Geometry: final body of the model. Coordinates: model frame, mm. Face numbers are marked on the shaded views. A direction names the side the tool comes from. Give positions to 0.01 mm unless a question says otherwise; leave off trailing zeros. Write each loop counter-clockwise with the first axis right and the second up, starting at its lowest first coordinate (ties: lowest second). Pieces come first, ordered by that corner, then holes. Notation, with made-up numbers: (-10.5, -15.5) -> (34.5, -15.5) arc R17 ccw to (34.5, -11.5) -> close; hole circle Ø2 at (-33.5, 19). An arc over 180 degrees is marked (long way). Answer as a JSON object with one key per item and string values. Group by question number.
(1) Section query D-D on z = 3.5. Output: boundary loops of the cut face in (x, y), plus the area to 3 significant figures.
(2) Section query A-A on x = 12.7. Output: boundary loops of the cut face in (y, z), plus the area to 3 significant figures.
(3) Draft query along Z for the marked faces 3, 4 and 5. Return one class per face: +Z half, -Z half, draft (parallel to the pull), parting line (faces both ways), or undercut.
(4) Material intervals for probe 1 along X at (y, z) = (0.75, 0); probe 2 along Z at (x, y) = (12.5, -6.5); probe 3 along Y at (x, z) = (18.25, 4.5), sorted ascending.
(5) Section query B-B on z = 0. Output: boundary loops of the cut face in (x, y), plus the area to 3 significant figures.
(6) Section query C-C on x = 2.75. Output: boundary loops of the cut face in (y, z).
(7) Contact query for flat-ended pins moving along their axis: pin 1 Ø5 at (x, z) = (13, 0) entering from +Y; pin 2 Ø3.5 at (x, z) = (12.7, 0) entering from -Y; pin 3 Ø0.6 at (y, z) = (7, 6.5) entering from -X; pin 4 Ø0.9 at (y, z) = (-0.5, -6.5) entering from -X. Output: stop coordinate, or through.
(8) Set-up query: the marked faces 1 and 2. Return all of +Z, -Z, +X, -X, +Y, -Y with unobstructed straight access to the full face (end or side cutting, diameter ignored); none if empty.
from build123d import *

# Parameters (mm, degrees)
SKETCH1_W           = 15
SKETCH1_H           = 15
BOSS_EXTRUDE1_DEPTH = 25.4
SKETCH2_R           = 2.75
CUT_EXTRUDE1_DEPTH  = 31.436984082
SKETCH3_W           = 10
SKETCH3_H           = 6.858
SKETCH3_R           = 1.5875
CUT_EXTRUDE2_DEPTH  = 1.778
FILLET1_R           = 0.79375
CUT_EXTRUDE3_DEPTH  = 0.5


with BuildPart() as part:
    # Sketch1 → Boss-Extrude1 (new body)
    with BuildSketch(Plane(origin=(0, 0, 0), x_dir=(0, 0, -1), z_dir=(1, 0, 0))):
        Rectangle(SKETCH1_W, SKETCH1_H)
    extrude(amount=BOSS_EXTRUDE1_DEPTH)

    # Sketch2 → Cut-Extrude1 (cut, through all)
    with BuildSketch(Plane(origin=(0, 7.5, 0), x_dir=(1, 0, 0), z_dir=(0, 1, 0))):
        with Locations(Location((12.7, 0, 0), (0, 0, 270))):
            Circle(SKETCH2_R)
    extrude(amount=-CUT_EXTRUDE1_DEPTH, mode=Mode.SUBTRACT)

    # Sketch3 → Cut-Extrude2 (cut)
    with BuildSketch(Plane(origin=(0, 0, -7.5), x_dir=(-1, 0, 0), z_dir=(0, 0, -1))):
        with Locations((-5, 0.071)):
            Rectangle(SKETCH3_W, SKETCH3_H)
        with Locations(Location((-4.92, 0.071, 0), (0, 0, 90))):
            Circle(SKETCH3_R, mode=Mode.SUBTRACT)
    extrude(amount=-CUT_EXTRUDE2_DEPTH, mode=Mode.SUBTRACT)

    # Fillet1
    fillet1_edges = [part.edges().sort_by_distance(p)[0] for p in [
        (10, -3.358, -6.611),
        (10, 3.5, -6.611),
    ]]
    fillet(fillet1_edges, radius=FILLET1_R)

    # Sketch7 → Cut-Extrude3 (cut)
    with BuildSketch(Plane(origin=(0, 7.5, 0), x_dir=(1, 0, 0), z_dir=(0, 1, 0))):
        Polygon((4, 7.5), (18.4, 7.5), (18.4, 5.5), (25.4, 5.5), (25.4, -5.5), (18.4, -5.5), (18.4, -7.5), (4, -7.5), (4, -5.5), (0, -5.5), (0, 5.5), (4, 5.5), align=None)
    extrude(amount=-CUT_EXTRUDE3_DEPTH, mode=Mode.SUBTRACT)


solid = part.part
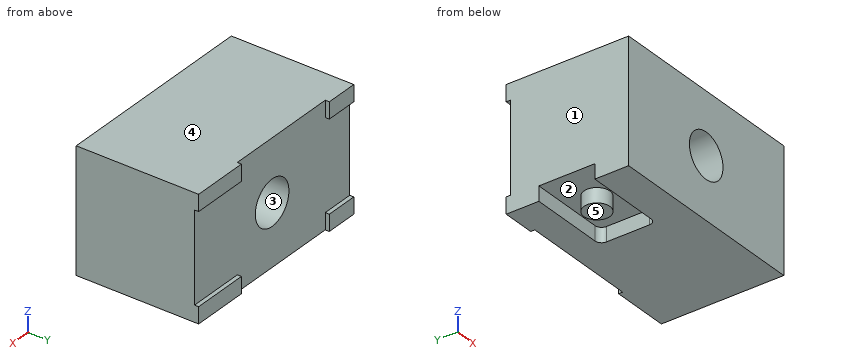
Answer list:
{
 "1": {"outline": "(0, -7.5) -> (25.4, -7.5) -> (25.4, 7) -> (0, 7) -> close", "area": "368 mm2"},
 "2": {"outline": "(-7.5, -7.5) -> (7, -7.5) -> (7, -2.75) -> (-7.5, -2.75) -> close; (-7.5, 2.75) -> (7, 2.75) -> (7, 7.5) -> (-7.5, 7.5) -> close", "area": "138 mm2"},
 "3": {"face 3": "undercut", "face 4": "+Z half", "face 5": "-Z half"},
 "4": {"probe 1": "0 to 9.95, 15.45 to 25.4", "probe 2": "-7.5 to -2.74, 2.74 to 7.5", "probe 3": "-7.5 to 7"},
 "5": {"outline": "(0, -7.5) -> (9.95, -7.5) -> (9.95, 7) -> (0, 7) -> close; (15.45, -7.5) -> (25.4, -7.5) -> (25.4, 7) -> (15.45, 7) -> close", "area": "289 mm2"},
 "6": {"outline": "(-7.5, -7.5) -> (-3.36, -7.5) -> (-3.36, -5.72) -> (3.5, -5.72) -> (3.5, -7.5) -> (7.5, -7.5) -> (7.5, -5.5) -> (7, -5.5) -> (7, 5.5) -> (7.5, 5.5) -> (7.5, 7.5) -> (-7.5, 7.5) -> close"},
 "7": {"pin 1": "y = 7", "pin 2": "through", "pin 3": "x = 0", "pin 4": "x = 3.34"},
 "8": {"face 1": "+Z, -Z, -X, +Y, -Y", "face 2": "-Z"}
}
